from build123d import *

# Parameters (mm, degrees)
PAD_DEPTH            = 20
SKETCH001_W          = 18
SKETCH001_H          = 16
POCKET_DEPTH         = 18.001
POCKET001_DEPTH      = 2.001
POCKET002_DEPTH      = 1
POCKET002_DEPTH_BACK = -5
POCKET003_DEPTH      = 2.001
POCKET004_DEPTH      = 1


with BuildPart() as part:
    # Sketch → Pad (new body)
    with BuildSketch(Plane.XY):
        Polygon((0, 0), (0, 20), (20, 0), align=None)
    extrude(amount=PAD_DEPTH)

    # Sketch001 → Pocket (cut, through all)
    with BuildSketch(Plane.XZ.offset(-2)):
        with Locations((11, 10)):
            Rectangle(SKETCH001_W, SKETCH001_H)
    extrude(amount=-POCKET_DEPTH, mode=Mode.SUBTRACT)

    # Sketch002 (on Face9 of Pocket) → Pocket001 (cut, through all)
    with BuildSketch(Plane.YZ.offset(2)):
        with BuildLine():
            ThreePointArc((4.8, 12.8), (2, 10), (4.8, 7.2))
            Line((4.8, 7.2), (15.2, 7.2))
            ThreePointArc((15.2, 7.2), (18, 10), (15.2, 12.8))
            Line((4.8, 12.8), (15.2, 12.8))
        make_face()
    extrude(amount=-POCKET001_DEPTH, mode=Mode.SUBTRACT)

    # Sketch003 (on Face13 of Pocket001) → Pocket002 (cut, two sides)
    with BuildSketch(Plane.YZ.offset(2)) as pocket002_sk:
        with BuildLine():
            ThreePointArc((15.2, 5.5), (19.7, 10), (15.2, 14.5))
            Line((4.8, 14.5), (15.2, 14.5))
            ThreePointArc((4.8, 14.5), (3.317186, 14.248678), (2, 13.522783))
            Line((2, 13.522783), (2, 6.477217))
            ThreePointArc((2, 6.477217), (3.317186, 5.751322), (4.8, 5.5))
            Line((4.8, 5.5), (15.2, 5.5))
        make_face()
    extrude(amount=-POCKET002_DEPTH, mode=Mode.SUBTRACT)
    extrude(pocket002_sk.sketch, amount=-POCKET002_DEPTH_BACK, mode=Mode.SUBTRACT)

    # Sketch004 (on Face21 of Pocket002) → Pocket003 (cut, through all)
    with BuildSketch(Plane(origin=(0, 2, 0), x_dir=(-1, 0, 0), z_dir=(0, 1, 0))):
        with BuildLine():
            ThreePointArc((-16.2, 11.8), (-18, 10), (-16.2, 8.2))
            Line((-16.2, 8.2), (-3.8, 8.2))
            ThreePointArc((-3.8, 8.2), (-2, 10), (-3.8, 11.8))
            Line((-16.2, 11.8), (-3.8, 11.8))
        make_face()
    extrude(amount=-POCKET003_DEPTH, mode=Mode.SUBTRACT)

    # Sketch005 (on Face15 of Pocket003) → Pocket004 (cut)
    with BuildSketch(Plane(origin=(0, 2, 0), x_dir=(-1, 0, 0), z_dir=(0, 1, 0))):
        with BuildLine():
            ThreePointArc((-16.2, 13), (-19.2, 10), (-16.2, 7))
            Line((-16.2, 7), (-3.8, 7))
            ThreePointArc((-3.8, 7), (-2.851317, 7.15395), (-2, 7.6))
            Line((-2, 12.4), (-2, 7.6))
            ThreePointArc((-2, 12.4), (-2.851317, 12.84605), (-3.8, 13))
            Line((-16.2, 13), (-3.8, 13))
        make_face()
    extrude(amount=-POCKET004_DEPTH, mode=Mode.SUBTRACT)


solid = part.part
The model under review builds one solid part; all positions refer to its coordinate system, in mm. A direction names the side the tool comes from. Coordinates: 2 decimals unless noted, no trailing zeros. Loops run counter-clockwise (first coordinate to the right, second up) from the corner with the lowest first, then second, coordinate; pieces in that order, holes last.
(1) Tool access review of faces 5 (the cylindrical face through (17.576, 1.507, 7.334)), 6 (the flat face through (0.5, 9.9, 7.2)), 7 (the flat face through (1, 10, 7)), 8 (the flat face through (8, 8, 2)), 9 (the flat face through (6, 6, 0)): name each direction out of +Z, -Z, +X, -X, +Y, -Y from which nothing blocks a thin tool from reaching the whole face with its end or side.
Determined:
face 5: +Y
face 6: +X, -X
face 7: +X
face 8: +X, +Y
face 9: -Z, +X, -X, +Y, -Y
(2) Draft analysis for pull direction X (two halves, no side actions). For faces 1 (the flat face through (1.5, 9.9, 14.5)), 2 (the cylindrical face through (18, 0.5, 10)), 3 (the flat face through (0, 10, 5)), 4 (the flat face through (10, 10, 19)), state which applies: +X half, -X half, draft (parallel to the pull), parting line (faces both ways), or undercut.
Determined:
face 1: draft
face 2: undercut
face 3: -X half
face 4: +X half
(3) Wall thickness on L1, parallel to Z at x = 11, y = 3.25; L2, parallel to Y at x = 15, z = 6; L3, parallel to Y at x = 3.75, z = 7.5: over which ranges is each line inside the solid? List them lowest first.
Determined:
L1: z = 0 to 2, 18 to 20
L2: y = 0 to 2
L3: y = 0 to 1
(4) Consider section C-C, the plane z = 10.75. Give the boundary of the cut face in (x, y), plus the area to 3 significant figures.
Determined:
outline: (0, 0) - (2.16, 0) - (2.16, 1) - (2, 1) - (2, 2) - (1, 2) - (1, 2.1) - (0, 2.1) - close; (0, 17.9) - (1, 17.9) - (1, 19) - (0, 20) - close; (17.84, 0) - (20, 0) - (19, 1) - (17.84, 1) - close
area: 7.53 mm2
(5) Insertion check: P1, Ø3, axis at y = 13.5, z = 8.5, coming from the -X side; P2, Ø7, axis at y = 8.5, z = 10.5, coming from the +X side; P3, Ø5, axis at x = 8, z = 13, coming from the +Y side; P4, Ø1.3, axis at y = 7, z = 4.5, coming from the +X side. Each pin has a flat end and moves straight along its axis. Give the tip position at first contact, or say it passes through.
Determined:
P1: stops at x = 0
P2: stops at x = 1
P3: stops at y = 2
P4: stops at x = 2
(6) Consider section D-D, the plane z = 5. Give the boundary of the cut face in (x, y).
Determined:
outline: (0, 0) - (20, 0) - (18, 2) - (2, 2) - (2, 18) - (0, 20) - close
(7) Consider section A-A, the plane y = 8.25. Give the boundary of the cut face in (x, z).
Determined:
outline: (0, 0) - (11.75, 0) - (11.75, 2) - (2, 2) - (2, 5.5) - (1, 5.5) - (1, 7.2) - (0, 7.2) - close; (0, 12.8) - (1, 12.8) - (1, 14.5) - (2, 14.5) - (2, 18) - (11.75, 18) - (11.75, 20) - (0, 20) - close
(8) Consider section B-B, the plane x = 10. Give the boundary of the cut face in (y, z).
Determined:
outline: (0, 0) - (10, 0) - (10, 2) - (2, 2) - (2, 7) - (1, 7) - (1, 8.2) - (0, 8.2) - close; (0, 11.8) - (1, 11.8) - (1, 13) - (2, 13) - (2, 18) - (10, 18) - (10, 20) - (0, 20) - close
